Source: CAD feature listing. Evaluate the final solid. Frame: model axes, mm. A direction names the side the tool comes from. Coordinates: 2 decimals unless noted, no trailing zeros. Loops run counter-clockwise (first coordinate to the right, second up) from the corner with the lowest first, then second, coordinate; pieces in that order, holes last.
```python
from build123d import *

# Parameters (mm, degrees)
F1_DEPTH = 12.5


with BuildPart() as f1:
    # F0 (on Front) → F1 (new body)
    with BuildSketch(Plane.XZ):
        with BuildLine():
            Line((4.907477, 8.5), (9.814955, 0))
            Line((9.814955, 0), (4.907477, -8.5))
            Line((4.907477, -8.5), (-4.907477, -8.5))
            Line((-4.907477, -8.5), (-9.814955, 0))
            Line((-9.814955, 0), (-5.47339, 7.51981))
            Line((-5.47339, 7.51981), (-6.011273, 8.456076))
            ThreePointArc((-6.011273, 8.456076), (5.168242, -8.996105), (-4.277084, 9.452363))
            Line((-4.277084, 9.452363), (-3.729954, 8.5))
            Line((-3.729954, 8.5), (4.907477, 8.5))
        make_face()
    extrude(amount=F1_DEPTH)


solid = f1.part
```
Q1. Reachability of faces 5 (the flat face through (8, 0, -4)), 6 (the flat face through (7.327, -6.162, 4.31)), 7 (the flat face through (1, -6, 8.5)) from +Z, -Z, +X, -X, +Y, -Y: full face, straight path, thin tool, end or side. Return the list, or none.
Q2. Section query D-D on z = -9. Return the cut outline in (x, y).
Q3. Section query B-B on x = 8.25. Return the cut outline in (y, z).
Q4. Section query A-A on z = -1.5. Return the cut outline in (x, y).
Q5. First-contact query: pin 1 Ø4 at (y, z) = (-3, -6.5) entering from +X; pin 2 Ø1.5 at (x, y) = (3.5, -11) entering from +Z; pin 3 Ø1.5 at (y, z) = (-7.5, -3.5) entering from +X; pin 4 Ø4.5 at (x, y) = (-1.5, -3.5) entering from -Z (3 decimals). Flat tips, straight axial feed; report the tip coordinate or a pass-through.
Q6. Material intervals for line 1 along Z through (x, y) = (-0.25, -4); line 2 along Z through (x, y) = (-7.5, -5.25); line 3 along X through (y, z) = (-7, 3.5), sorted ascending.
Q7. Draft query along X for faces 1 (the flat face through (8, -12.5, -4)), 2 (the flat face through (-4.007, -6.162, 8.983)), 3 (the cylindrical face through (4.8, -6.2, -9.2)), 4 (the flat face through (-5.74, -6.16, 7.98)). Return one class per face: released by +X, released by -X, zero draft, split by the parting line, or undercut.
Q8. Section query C-C on y = -3. Return the cut outline in (x, z) (3 decimals).
Resolved:
1. face 5: +Z, -Z, +X, -X, +Y
1. face 6: +Y, -Y
1. face 7: -X, +Y, -Y
2. outline: (-5.16, -12.5) - (5.16, -12.5) - (5.16, 0) - (-5.16, 0) - close
3. outline: (-12.5, -6.29) - (0, -6.29) - (0, -2.71) - (-12.5, -2.71) - close; (-12.5, 2.71) - (0, 2.71) - (0, 6.29) - (-12.5, 6.29) - close
4. outline: (-10.27, -12.5) - (-8.95, -12.5) - (-8.95, 0) - (-10.27, 0) - close; (8.95, -12.5) - (10.27, -12.5) - (10.27, 0) - (8.95, 0) - close
5. pin 1: stops at x = 9.35
5. pin 2: stops at z = 10
5. pin 3: stops at x = 10
5. pin 4: stops at z = -10.375
6. line 1: z = -10.37 to -8.5, 8.5 to 10.37
6. line 2: z = -7.17 to -4.01, 4.01 to 7.17
6. line 3: x = -9.77 to -7.79, 7.79 to 9.77
7. face 1: zero draft
7. face 2: released by -X
7. face 3: split by the parting line
7. face 4: undercut
8. outline: (-9.815, 0) - (-5.473, 7.52) - (-6.011, 8.456) arc R10.375 ccw (long way) to (-4.277, 9.452) - (-3.73, 8.5) - (4.907, 8.5) - (9.815, 0) - (4.907, -8.5) - (-4.907, -8.5) - close
